Geometry: see drawing. Coordinates: mm, zero at the bounding-box minimum. A direction names the side the tool comes from. Give positions to 0.01 mm unless a question says otherwise; leave off trailing zeros. Write each loop counter-clockwise with the first axis right and the second up, starting at its lowest first coordinate (ties: lowest second). Pieces come first, ordered by that corner, then holes. Notation, with made-up numbers: (14, -19) - (48, -19) arc R13 ccw to (48, -12) - close; hole circle Ø4 at (49.5, -5). An arc over 180 degrees is marked (long way). Use CSV: the item, a comma, the result in double quotes. Start each with the question number.
(1) Section B-B on z = 3.5. Output: boundary loops of the cut face in (x, y), and give its area (3 significant figures).
(2) Section A-A on y = 3.5. Output: boundary loops of the cut face in (x, z).
(3) Draft query along Y for the marked faces 3, 4 and 5. Return one class per face: released by +Y, released by -Y, zero draft, split by the parting line, or undercut.
(4) Line query: probe 1 along Y at (x, z) = (8.5, 3); probe 2 along Z at (x, y) = (8.25, 4); probe 3 along Y at (x, z) = (8, 1.75). Output: solid intervals per line, ascending. Write a range as [from, to].
(5) Section D-D on y = 5.75. Output: boundary loops of the cut face in (x, z), and give its area (3 significant figures).
(6) First-contact query: pin 1 Ø1 at (x, z) = (5, 1.5) entering from +Y; pin 2 Ø1.5 at (x, y) = (3.5, 4.5) entering from -Z; pin 3 Ø3 at (x, y) = (4.5, 6) entering from -Z. Flat tips, straight axial feed; report the tip coordinate or a pass-through.
(7) Reachability of the marked faces 1 and 2 from +Z, -Z, +X, -X, +Y, -Y: full face, straight path, thin tool, end or side. Return the list, or none.
(8) Section C-C on x = 7.25. Output: boundary loops of the cut face in (y, z).
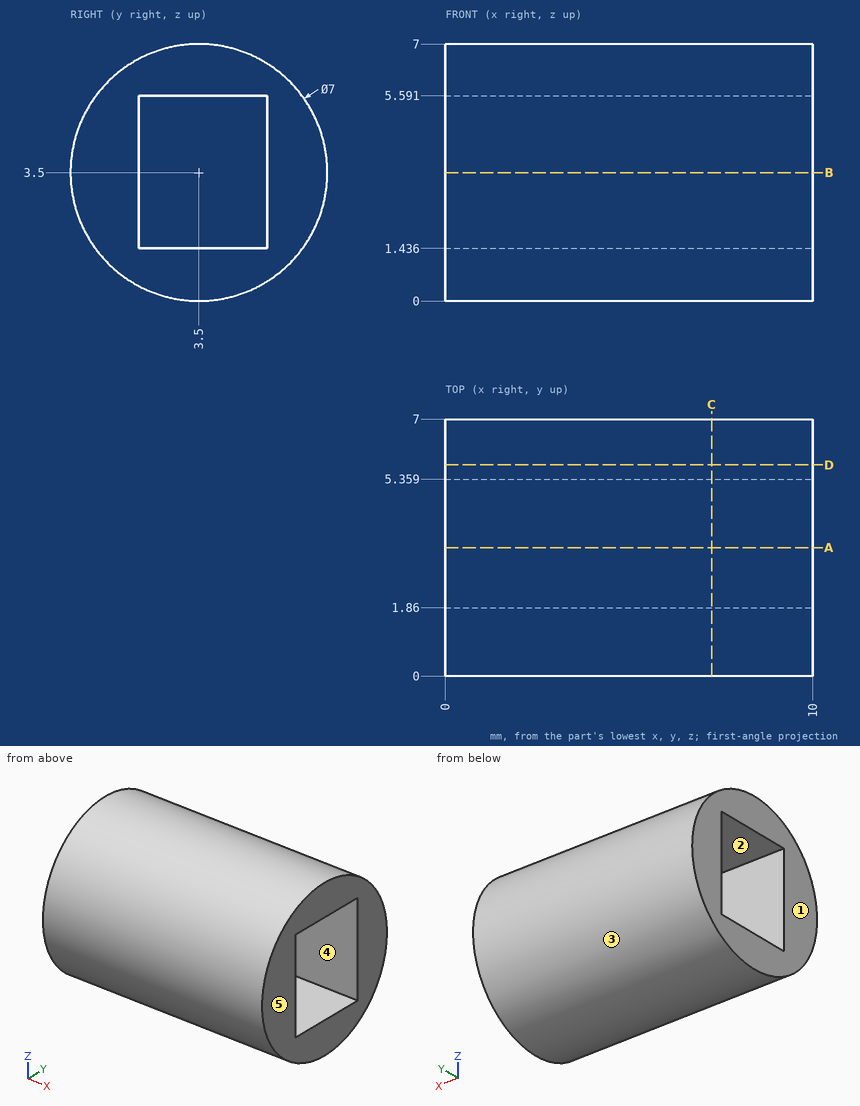
Check values:
1,outline,"(0, 0) - (10, 0) - (10, 1.86) - (0, 1.86) - close; (0, 5.36) - (10, 5.36) - (10, 7) - (0, 7) - close"
1,area,"35.0 mm²"
2,outline,"(0, 0) - (10, 0) - (10, 1.44) - (0, 1.44) - close; (0, 5.59) - (10, 5.59) - (10, 7) - (0, 7) - close"
3,face 3,"split by the parting line"
3,face 4,"undercut"
3,face 5,"zero draft"
4,probe 1,"y = [0.04, 1.86], [5.36, 6.96]"
4,probe 2,"z = [0.04, 1.44], [5.59, 6.96]"
4,probe 3,"y = [0.47, 1.86], [5.36, 6.53]"
5,outline,"(0, 0.82) - (10, 0.82) - (10, 6.18) - (0, 6.18) - close"
5,area,"53.6 mm²"
6,pin 1,"stops at y = 6.66"
6,pin 2,"stops at z = 0.01"
6,pin 3,"stops at z = 0.15"
7,face 1,"+Z, -Z, -X, +Y, -Y"
7,face 2,"+X, -X"
8,outline,"circle Ø7 at (3.5, 3.5); hole (1.86, 1.44) - (5.36, 1.44) - (5.36, 5.59) - (1.86, 5.59) - close"
